```python
from build123d import *

# Parameters (mm, degrees)
BOSS_EXTRUDE2_START     = 5.5
SKETCH8_R               = 2
BOSS_EXTRUDE2_DEPTH     = 5.5
SKETCH9_R               = 2.05
CUT_EXTRUDE3_DEPTH      = 5.5
CUT_EXTRUDE4_DEPTH      = 5.5
CUT_EXTRUDE4_DEPTH_BACK = 3
SKETCH10_R              = 0.75
SKETCH12_R              = 2.032145481
CUT_EXTRUDE5_DEPTH      = 1.2
CUT_EXTRUDE11_START     = -3
SKETCH15_R              = 1.5
CUT_EXTRUDE11_DEPTH     = 21.2
CUT_EXTRUDE12_START     = 24.2
SKETCH16_R              = 1.5
CUT_EXTRUDE12_DEPTH     = 21.2
SKETCH17_W              = 12.094428853
SKETCH17_H              = 12.59473796
CUT_EXTRUDE14_DEPTH     = 21.2
SKETCH18_R              = 5.596164195
CUT_EXTRUDE15_DEPTH     = 0.75


with BuildPart() as part:
    # Sketch1 → Revolve2 (revolve)
    with BuildSketch(Plane.XY):
        Polygon((-0.75, -3.5), (-0.75, -2), (-2, -2), (-2, 3.5), (-4, 3.5), (-4, -3.5), align=None)
        Polygon((2, -2), (0.75, -2), (0.75, -3.5), (4, -3.5), (4, 3.5), (2, 3.5), align=None)
    revolve(axis=Axis((0, 0, 0), (0, -1, 0)))

    # Sketch8 → Boss-Extrude2 (add)
    with BuildSketch(Plane(origin=(0, -2, 0), x_dir=(1, 0, 0), z_dir=(0, 1, 0)).offset(BOSS_EXTRUDE2_START)):
        Circle(SKETCH8_R)
    extrude(amount=-BOSS_EXTRUDE2_DEPTH)

    # Sketch9 → Cut-Extrude3 (cut)
    with BuildSketch(Plane.XZ.offset(2)):
        Circle(SKETCH9_R)
    extrude(amount=-CUT_EXTRUDE3_DEPTH, mode=Mode.SUBTRACT)

    # Sketch10 → Cut-Extrude4 (cut, two sides: drawn at the far end of the back side and taken through both)
    with BuildSketch(Plane.XY.offset(-CUT_EXTRUDE4_DEPTH_BACK)):
        with Locations(Location((2.513623539, 0, 0), (0, 0, 180))):
            Circle(SKETCH10_R)
        with Locations(Location((-2.513623539, 0, 0), (0, 0, 180))):
            Circle(SKETCH10_R)
    extrude(amount=CUT_EXTRUDE4_DEPTH + CUT_EXTRUDE4_DEPTH_BACK, mode=Mode.SUBTRACT)

    # Sketch12 → Cut-Extrude5 (cut)
    with BuildSketch(Plane(origin=(0, -2, 0), x_dir=(1, 0, 0), z_dir=(0, 1, 0))):
        Circle(SKETCH12_R)
    extrude(amount=CUT_EXTRUDE5_DEPTH, mode=Mode.SUBTRACT)

    # Sketch15 → Cut-Extrude11 (cut)
    with BuildSketch(Plane.XY.offset(CUT_EXTRUDE11_START)):
        with Locations((2.513623539, 0)):
            Circle(SKETCH15_R)
        with Locations((-2.513623539, 0)):
            Circle(SKETCH15_R)
    extrude(amount=-CUT_EXTRUDE11_DEPTH, mode=Mode.SUBTRACT)

    # Sketch16 → Cut-Extrude12 (cut)
    with BuildSketch(Plane.XY.offset(CUT_EXTRUDE12_START)):
        with Locations((2.513623539, 0)):
            Circle(SKETCH16_R)
        with Locations((-2.513623539, 0)):
            Circle(SKETCH16_R)
    extrude(amount=-CUT_EXTRUDE12_DEPTH, mode=Mode.SUBTRACT)

    # Sketch17 → Cut-Extrude14 (cut)
    with BuildSketch(Plane.XY):
        with Locations((-0.435051398, -0.913607935)):
            Rectangle(SKETCH17_W, SKETCH17_H)
    extrude(amount=-CUT_EXTRUDE14_DEPTH, mode=Mode.SUBTRACT)

    # Sketch18 → Cut-Extrude15 (cut)
    with BuildSketch(Plane.XZ.offset(3.5)):
        Circle(SKETCH18_R)
    extrude(amount=-CUT_EXTRUDE15_DEPTH, mode=Mode.SUBTRACT)


solid = part.part
```
Verification items for the finished model (mm, model axes). A direction names the side the tool comes from. Coordinates: 2 decimals unless noted, no trailing zeros. Loops run counter-clockwise (first coordinate to the right, second up) from the corner with the lowest first, then second, coordinate; pieces in that order, holes last. Notation, with made-up numbers: (52.25, 35) - (82.25, 35) arc R16 ccw to (82.25, 40) - close; hole circle Ø8 at (10.25, 17). An arc over 180 degrees is marked (long way). Answer as a JSON object with one key per item and string values.
(1) Go/stop test with flat-tipped pins: pin 1 Ø1.5 at (y, z) = (-1.5, 2.5) entering from -X; pin 2 Ø0.6 at (x, z) = (0.5, 1.5) entering from +Y; pin 3 Ø2 at (x, y) = (-2.51, 0) entering from -Z; pin 4 Ø2 at (y, z) = (-1, 3.5) entering from +X. Record where each tip stops, or that it passes through.
Response:
{"pin 1": "stops at x = -3.6", "pin 2": "stops at y = -2", "pin 3": "stops at z = 0", "pin 4": "stops at x = 3.12"}
(2) Scan lines: line 1 along Y through (x, z) = (2.5, 1); line 2 along Y through (x, z) = (1.5, 0.2); line 3 along Z through (x, y) = (0, 1.75). Record each from-to range of solid material in increasing order.
Response:
{"line 1": "y = -2.75 to -0.75, 0.75 to 3.5", "line 2": "y = -2.75 to -2", "line 3": "z = 2.05 to 4"}
(3) Access from +Z, -Z, +X, -X, +Y, -Y to the whole of each face (thin tool, end or side, straight path). Record for faces 5 (the cylindrical face through (0.05, 0.71, 2.05)), 6 (the flat face through (-1.5, 0, 3)), 7 (the flat face through (1.6, 0, 3)).
Response:
{"face 5": "-Z, +Y", "face 6": "+Z, -X", "face 7": "+Z, +X"}
(4) Cross-section at B-B, the plane y = 0. Record the boundary of the cut face in (x, z).
Response:
{"outline": "(-4, 0) - (-3.26, 0) - (-3.26, 2.31) arc R4 ccw to start; (-1.76, 1.05) arc R2.05 cw to (1.76, 1.05) - (1.76, 3) - (1.01, 3) - (1.01, 3.87) arc R4 ccw to (-1.01, 3.87) - (-1.01, 3) - (-1.76, 3) - close; (3.26, 0) - (4, 0) arc R4 ccw to (3.26, 2.31) - close"}
(5) Cross-section at D-D, the plane x = 0. Record the boundary of the cut face in (y, z), then the cut area to 3 significant figures.
Response:
{"outline": "(-2.75, 0.75) - (-2, 0.75) - (-2, 2.05) - (3.5, 2.05) - (3.5, 4) - (-2.75, 4) - close", "area": "13.2 mm²"}
(6) Mould release check, pull along X, two halves, no side actions. Record for faces 1 (the flat face through (-0.1, 3.5, 2.4)), 2 (the flat face through (0, -2, 1)), 3 (the cylindrical face through (3.263, -0.033, 1.479)), 4 (the cylindrical face through (0, 0, 4)): pulls with the +X half, pulls with the -X half, needs draft (parallel to the pull), parting line crosses it, or undercut.
Response:
{"face 1": "needs draft", "face 2": "undercut", "face 3": "undercut", "face 4": "parting line crosses it"}
(7) Cross-section at A-A, the plane x = -2.75. Record the boundary of the cut face in (y, z).
Response:
{"outline": "(-2.75, 0) - (-0.71, 0) - (-0.71, 2.9) - (-2.75, 2.9) - close; (0.71, 0) - (3.5, 0) - (3.5, 2.9) - (0.71, 2.9) - close"}
(8) Cross-section at C-C, the plane z = 1.8. Record the boundary of the cut face in (x, y).
Response:
{"outline": "(-3.57, -2.75) - (3.57, -2.75) - (3.57, 3.5) - (0.98, 3.5) - (0.98, -2) - (-0.98, -2) - (-0.98, 3.5) - (-3.57, 3.5) - close; hole circle Ø1.5 at (-2.51, 0); hole circle Ø1.5 at (2.51, 0)"}
